Could you check a few things on this model? Use its own coordinates, in mm. Round coordinates to 2 decimals unless told otherwise and drop trailing zeros. Order: outer loops, then holes, each group sorted by start corner. A loop starts at its lowest first (then second) coordinate and runs counter-clockwise, first axis right, second up. Notation, with made-up numbers: (-35.75, 70) - (-21.75, 70) arc R21 cw to (-21.75, 101) - close; hole circle Ø5 at (-25, -39.5). An arc over 180 degrees is marked (long way). Use one line per item in the form item = value.
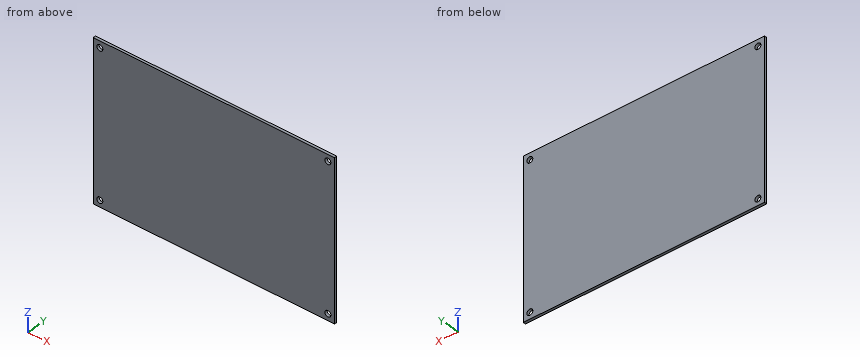
from build123d import *

# Parameters (mm, degrees)
SKETCH2_W           = 146.5
SKETCH2_H           = 95
SKETCH2_R           = 1.8
BOSS_EXTRUDE1_DEPTH = 1.6


with BuildPart() as part:
    # Sketch2 → Boss-Extrude1 (new body)
    with BuildSketch(Plane(origin=(0, 0, 0), x_dir=(1, 0, 0), z_dir=(0, 1, 0))):
        Rectangle(SKETCH2_W, SKETCH2_H)
        with Locations((-69.25, 43.5)):
            Circle(SKETCH2_R, mode=Mode.SUBTRACT)
        with Locations((69.25, 43.5)):
            Circle(SKETCH2_R, mode=Mode.SUBTRACT)
        with Locations((69.25, -43.5)):
            Circle(SKETCH2_R, mode=Mode.SUBTRACT)
        with Locations((-69.25, -43.5)):
            Circle(SKETCH2_R, mode=Mode.SUBTRACT)
    extrude(amount=-BOSS_EXTRUDE1_DEPTH)


solid = part.part
Item 1: Will these pins go through, and if not, where does the flat tip stop? P1, Ø3, axis at x = 69.25, z = -43.5, coming from the +Y side; P2, Ø8, axis at x = -19.5, z = -8.5, coming from the +Y side.
Found:
P1 = through
P2 = 0
Item 2: I need wall thicknesses on L1, parallel to X at y = -1.15, z = -43.5; L2, parallel to Z at x = -69.25, y = -0.95. Which ranges of each line are inside material? Lowest first, please.
Found:
L1 = -73.25 to -71.05, -67.45 to 67.45, 71.05 to 73.25
L2 = -47.5 to -45.3, -41.7 to 41.7, 45.3 to 47.5
Item 3: Imagine slicing it at B-B on z = 43.5. Please give me the cut outline in (x, y).
Found:
outline = (-73.25, -1.6) - (-71.05, -1.6) - (-71.05, 0) - (-73.25, 0) - close; (-67.45, -1.6) - (67.45, -1.6) - (67.45, 0) - (-67.45, 0) - close; (71.05, -1.6) - (73.25, -1.6) - (73.25, 0) - (71.05, 0) - close
Item 4: Imagine slicing it at A-A on x = 69.25. Please give me the cut outline in (y, z), plus the area to 3 significant figures.
Found:
outline = (-1.6, -47.5) - (0, -47.5) - (0, -45.3) - (-1.6, -45.3) - close; (-1.6, -41.7) - (0, -41.7) - (0, 41.7) - (-1.6, 41.7) - close; (-1.6, 45.3) - (0, 45.3) - (0, 47.5) - (-1.6, 47.5) - close
area = 140 mm2
